Geometry: final body of the model. Coordinates: model frame, mm. Coordinates: 2 decimals unless noted, no trailing zeros. Write each loop counter-clockwise with the first axis right and the second up, starting at its lowest first coordinate (ties: lowest second). Pieces come first, ordered by that corner, then holes. Notation, with made-up numbers: (-23, 8.5) - (-14, 8.5) arc R18 cw to (-14, 39.5) - close; hole circle Ø2 at (38.25, 82.25). An arc over 180 degrees is marked (long way). Put each result on its own line as item: value.
Autodesk Inventor part; units mm, degrees
ref_plane "YZ Plane" through (0, 0, 0) normal (1, 0, 0) x (0, 1, 0)
ref_plane "XZ Plane" through (0, 0, 0) normal (0, 1, 0) x (-1, 0, 0)
ref_plane "XY Plane" through (0, 0, 0) normal (0, 0, 1) x (1, 0, 0)
sketch "Náčrt2" plane through (0, 0, 0) normal (0, 1, 0) x (-1, 0, 0)
  line L0 (11.5, 17.5) -> (-11.5, 17.5) construction
  line L1 (-17.5, 11.5) -> (-17.5, -11.5) construction
  line L2 (-11.5, -17.5) -> (11.5, -17.5) construction
  line L3 (17.5, -11.5) -> (17.5, 11.5) construction
  line L4 (42.5, 36) -> (42.5, -77.5) construction
  line L5 (9, -22.5) -> (-14, -22.5) construction
  line L6 (-20, -28.5) -> (-20, -51.5) construction
  line L7 (-14, -57.5) -> (9, -57.5) construction
  line L8 (15, -51.5) -> (15, -28.5) construction
  arc A0 (15, -28.5) -> (9, -22.5) centre (9, -28.5) ccw construction
  arc A1 (9, -57.5) -> (15, -51.5) centre (9, -51.5) ccw construction
  arc A2 (-20, -51.5) -> (-14, -57.5) centre (-14, -51.5) ccw construction
  arc A3 (-14, -22.5) -> (-20, -28.5) centre (-14, -28.5) ccw construction
  line L9 (-45.6938, -20) -> (9, -20) construction
  arc A4 (17.5, -28.5) -> (9, -20) centre (9, -28.5) ccw construction
  line L10 (17.5, -28.5) -> (17.5, -51.5) construction
  line L11 (17.5, -51.5) -> (15, -51.5) construction
  line L12 (-14, -22.5) -> (-45.6938, -22.5) construction
  line L13 (-45.6938, -22.5) -> (-45.6938, -20) construction
  arc A5 (17.5, 11.5) -> (11.5, 17.5) centre (11.5, 11.5) ccw construction
  arc A6 (11.5, -17.5) -> (17.5, -11.5) centre (11.5, -11.5) ccw construction
  arc A7 (-17.5, -11.5) -> (-11.5, -17.5) centre (-11.5, -11.5) ccw construction
  arc A8 (-11.5, 17.5) -> (-17.5, 11.5) centre (-11.5, 11.5) ccw construction
  line L14 (-11.5, -20) -> (11.5, -20) construction
  line L15 (-20, 73.4113) -> (-20, -11.5) construction
  arc A9 (-20, -11.5) -> (-11.5, -20) centre (-11.5, -11.5) ccw construction
  line L16 (-17.5, 11.5) -> (-17.5, 73.4113) construction
  line L17 (-17.5, 73.4113) -> (-20, 73.4113) construction
  line L18 (11.5, -20) -> (11.5, -17.5) construction
  line L19 (17.5, 17.5) -> (-17.5, 17.5) construction
  line L20 (-17.5, 17.5) -> (-17.5, 52.5) construction
  line L21 (-17.5, 52.5) -> (17.5, 52.5) construction
  line L22 (17.5, 52.5) -> (17.5, 17.5) construction
  circle A10 centre (0, 35) radius 6.5
  arc A11 (0, 51) -> (0, 19) centre (0, 35) ccw construction
  line L23 (0, 51) -> (27.5, 51) construction
  line L24 (0, 19) -> (11.5, 19) construction
  line L25 (27.5, 51) -> (42.5, 36) construction
  arc A12 (17.5, 13) -> (11.5, 19) centre (11.5, 13) ccw construction
  line L26 (17.5, 13) -> (17.5, -51.5) construction
  line L27 (-13.5, -57.5) -> (-13.5, -59.2574) construction
  line L28 (-12.6213, -61.3787) -> (14.1066, -88.1066) construction
  line L29 (24.7132, -92.5) -> (27.5, -92.5) construction
  arc A13 (27.5, -92.5) -> (42.5, -77.5) centre (27.5, -77.5) ccw construction
  arc A14 (14.1066, -88.1066) -> (24.7132, -92.5) centre (24.7132, -77.5) ccw construction
  arc A15 (-13.5, -59.2574) -> (-12.6213, -61.3787) centre (-10.5, -59.2574) ccw construction
  line L30 (17.5, -51.5) -> (17.5, -51.5) construction
  line L31 (6.4677, -58.2408) -> (-10.5, -57.5) construction
  line L32 (-13.5, -57.5) -> (-10.5, -57.5) construction
  line L33 (6.4677, -58.2408) -> (6.5, -57.5) construction
  line L34 (6.5, -57.5) -> (11.5, -57.5) construction
  arc A16 (11.5, -57.5) -> (17.5, -51.5) centre (11.5, -51.5) ccw construction
  arc A17 (-16, 35) -> (16, 35) centre (0, 35) ccw
  line L35 (16, 35) -> (16, 375)
  line L36 (-16, 35) -> (-16, 375)
  line L37 (6, 385) -> (-6, 385)
  arc A18 (16, 375) -> (6, 385) centre (6, 375) ccw
  arc A19 (-6, 385) -> (-16, 375) centre (-6, 375) ccw
  point P0 (0, 0)
  point P1 (17.5, 0)
  point P2 (0, 17.5)
  point P3 (42.5, 51)
  point P4 (17.5, 35)
  point P5 (0, 52.5)
  point P6 (-13.5, -60.5)
  dimension "d34" = 35
  dimension "d35" = 6
  dimension "d36" = 5
  dimension "d37" = 2.5
  dimension "d38" = 2.5
  dimension "d39" = 6
  dimension "d40" = 2.5
  dimension "d43" = 25
  dimension "d46" = 13
  dimension "d47" = 32
  dimension "d48" = 15
  dimension "d49" = 15
  dimension "d50" = 6
  dimension "d51" = 35
  dimension "d55" = 3
  dimension "d56" = 15
  dimension "d57" = 15
  dimension "d58" = 3
  dimension "d60" = 35
  dimension "d61" = 3
  dimension "d62" = 2.5
  dimension "d63" = 35
  dimension "d64" = 45
  dimension "d66" = 31
  dimension "d69" = 6
  dimension "d72" = 2.5
  dimension "d73" = 350
  dimension "d74" = 10
extrude "Vysunutí1" add sketch "Náčrt2" along normal blind 6
sketch "Náčrt5" plane through (0, 0, 0) normal (0, -1, 0) x (1, 0, 0)
  circle A0 centre (0, 35) radius 6.5
  arc A1 (-16, 35) -> (16, 35) centre (0, 35) ccw
  line L0 (16, 375) -> (16, 35)
  arc A2 (16, 375) -> (6, 385) centre (6, 375) ccw
  line L1 (-6, 385) -> (6, 385)
  arc A3 (-6, 385) -> (-16, 375) centre (-6, 375) ccw
  line L2 (-16, 35) -> (-16, 375)
  circle A4 centre (0, 305) radius 5
  point P0 (0, 0)
  point P1 (0, 385)
  dimension "d75" = 10
  dimension "d76" = 80
extrude "Vysunutí3" cut sketch "Náčrt5" against normal blind 10 contours A4
equation "\"PoloměrOhybu\" = Tloušťka"
equation "\"ŠířkaVýštipu\" = Tloušťka"
equation "\"HloubkaVýštipu\" = 0.5 * Tloušťka"
equation "\"VelikostRohovéhoVýštipu\" = 4 * Tloušťka"
equation "\"MinimálníZbytek\" = 2 * Tloušťka"
equation "\"PřechodovýPoloměr\" = PoloměrOhybu"
equation "\"VelikostJacobihoPoloměru\" = PoloměrOhybu"
equation "\"VelikostMezery\" = Tloušťka"
properties part number "DD_KVD_002_09" material "Nerezová ocel"
1. Section query C-C (y = 4.25). Return loops of the section in (x, z), then the cut area to 3 significant figures.
Answer below:
outline: (-16, 35) arc R16 ccw to (16, 35) - (16, 375) arc R10 ccw to (6, 385) - (-6, 385) arc R10 ccw to (-16, 375) - close; hole circle Ø13 at (0, 35); hole circle Ø10 at (0, 305)
area: 11,300 mm²
2. Section query B-B (x = 0). Return loops of the section in (y, z).
Answer below:
outline: (0, 19) - (6, 19) - (6, 28.5) - (0, 28.5) - close; (0, 41.5) - (6, 41.5) - (6, 300) - (0, 300) - close; (0, 310) - (6, 310) - (6, 385) - (0, 385) - close
3. Mould query, pull axis Z, two halves, no side actions, for faces 1 (the cylindrical face through (-0.651, 2.958, 309.957)), 2 (the cylindrical face through (0, 3, 19)), 3 (the cylindrical face through (13.15, 2.96, 381.99)), 4 (the cylindrical face through (0.846, 2.958, 28.555)). Classes: +Z half, -Z half, draft (parallel to the pull), parting line (faces both ways), or undercut.
Answer below:
face 1: undercut
face 2: -Z half
face 3: +Z half
face 4: undercut
4. Pin query (flat end, axial travel): pin 1 Ø3 at (x, y) = (10, 3.5) entering from +Z. Return the tip coordinate at first contact, or that it passes through.
Answer below:
pin 1: stops at z = 384.68
5. Ray query, probe 1 along Z at (x, y) = (0, 2.3); probe 2 along X at (y, z) = (1.75, 305); probe 3 along Z at (x, y) = (-2, 5.5). Return the intervals inside material, ascending. Write a range as from..to.
Answer below:
probe 1: z = 19..28.5, 41.5..300, 310..385
probe 2: x = -16..-5, 5..16
probe 3: z = 19.13..28.82, 41.18..300.42, 309.58..385
6. Section query A-A (z = 305). Return loops of the section in (x, y).
Answer below:
outline: (-16, 0) - (-5, 0) - (-5, 6) - (-16, 6) - close; (5, 0) - (16, 0) - (16, 6) - (5, 6) - close
